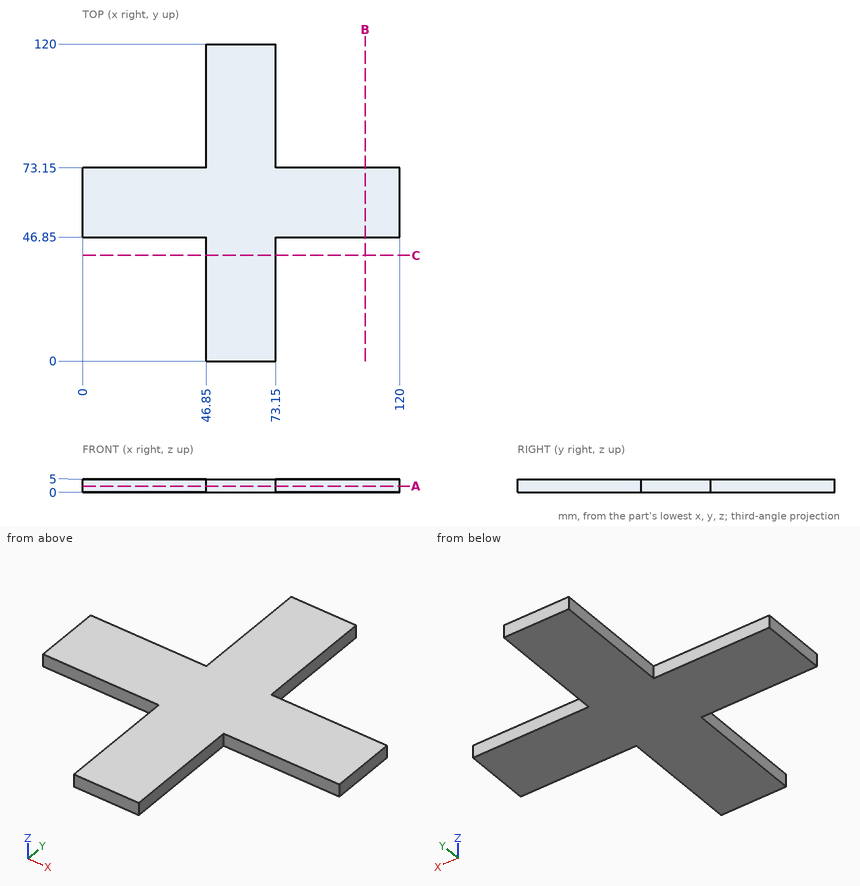
Answer from the drawing. Dimensions are ordinates in mm from the lowest x, y and z of the part. Coordinates: 2 decimals unless noted, no trailing zeros. Write each loop counter-clockwise with the first axis right and the second up, starting at its lowest first coordinate (ties: lowest second). Pieces come first, ordered by that corner, then holes. Notation, with made-up numbers: (-35, 89.25) - (-14, 89.25) arc R20 cw to (-14, 114.25) - close; hole circle Ø3 at (76.25, 5). An arc over 180 degrees is marked (long way). Answer as CSV lines item,"result".
1. Given P1, Ø2, axis at y = 108, z = 0.5, coming from the +X side; P2, Ø10, axis at x = 105, y = 56, coming from the -Z side; P3, Ø1.5, axis at x = 101.5, z = 1.5, coming from the +Y side, each flat-ended and moving along its own axis, determine where each tip first touches the part or whether it passes through.
Computed values:
P1,"stops at x = 73.15"
P2,"stops at z = 0"
P3,"stops at y = 73.15"
2. Find section B-B (x = 107). Give the vertices of the cut face in (y, z).
Computed values:
outline,"(46.85, 0) - (73.15, 0) - (73.15, 5) - (46.85, 5) - close"
3. Find section A-A (z = 2.3). Give the vertices of the cut face in (x, y).
Computed values:
outline,"(0, 46.85) - (46.85, 46.85) - (46.85, 0) - (73.15, 0) - (73.15, 46.85) - (120, 46.85) - (120, 73.15) - (73.15, 73.15) - (73.15, 120) - (46.85, 120) - (46.85, 73.15) - (0, 73.15) - close"
4. A straight line is drawn through the part: line 1 (X direction, y = 95.5, z = 3.85). Find the intervals that lie inside material, in ascending order. Write a range as [from, to].
Computed values:
line 1,"x = [46.85, 73.15]"
